Work out the finished part from the listing and answer in its coordinate system (mm). Round coordinates to 2 decimals unless told otherwise and drop trailing zeros. Loops run counter-clockwise (first coordinate to the right, second up) from the corner with the lowest first, then second, coordinate; pieces in that order, holes last. Notation, with made-up numbers: (8, 45) - (20, 45) arc R15 cw to (20, 66) - close; hole circle Ø1 at (72.25, 87). An arc over 180 degrees is marked (long way). Return JSON: item names as keys, results as strings.
from build123d import *

# Parameters (mm, degrees)
SKETCH1_R           = 4.2
BOSS_EXTRUDE1_DEPTH = 6.35


with BuildPart() as part:
    # Sketch1 → Boss-Extrude1 (new body)
    with BuildSketch(Plane(origin=(71.29240007, 0, 0), x_dir=(0, 0, -1), z_dir=(1, 0, 0))):
        with BuildLine():
            Line((916.713582015, 360.677443288), (922.204212824, 345.758563031))
            Line((922.204212824, 345.758563031), (895.973808013, 345.904541612))
            Line((895.973808013, 345.904541612), (897.39332308, 358.356278755))
            ThreePointArc((897.39332308, 358.356278755), (906.13613116, 367.152203744), (916.713582015, 360.677443288))
        make_face()
        with Locations((907.328968128, 357.223601629)):
            Circle(SKETCH1_R, mode=Mode.SUBTRACT)
    extrude(amount=BOSS_EXTRUDE1_DEPTH)


solid = part.part
1) Determine the mould class of faces 1 (the cylindrical face through (74.42, 353.5, -909.27)), 2 (the flat face through (74.42, 353.32, -919.42)), 3 (the flat face through (71.292, 352, -906)) for opening direction Y: pulls with the +Y half, pulls with the -Y half, needs draft (parallel to the pull), parting line crosses it, or undercut.
Verdict:
{"face 1": "undercut", "face 2": "pulls with the +Y half", "face 3": "needs draft"}
2) Flat-ended cylindrical pins translate along their axes: pin 1 (1 mm diameter, centred on x = 76, z = -908.5, fed in from +Y); pin 2 (1 mm diameter, centred on x = 72.5, y = 351, fed in from -Z); pin 3 (1 mm diameter, centred on x = 74, y = 355.5, fed in from +Z). Find the tip coordinate at first contact, or state that the pin passes through.
Verdict:
{"pin 1": "stops at y = 367.2", "pin 2": "stops at z = -920.46", "pin 3": "stops at z = -897.01"}
3) Section B-B (z = -906) is taken. Give the vertices of the cut face in (x, y).
Verdict:
{"outline": "(71.29, 345.85) - (77.64, 345.85) - (77.64, 353.24) - (71.29, 353.24) - close; (71.29, 361.21) - (77.64, 361.21) - (77.64, 367.13) - (71.29, 367.13) - close"}
4) Section C-C (x = 77.25) is taken. Give the vertices of the cut face in (y, z), and give its area (3 significant figures).
Verdict:
{"outline": "(345.76, -922.2) - (360.68, -916.71) arc R10 ccw to (358.36, -897.39) - (345.9, -895.97) - close; hole circle Ø8.4 at (357.22, -907.33)", "area": "370 mm2"}
5) Section D-D (y = 349.5) is taken. Give the vertices of the cut face in (x, z).
Verdict:
{"outline": "(71.29, -920.83) - (77.64, -920.83) - (77.64, -896.38) - (71.29, -896.38) - close"}
6) Find the intervals of material crossed by L1, parallel to Z at x = 75.5, y = 356.75; L2, parallel to Y at x = 73.25, z = -909; L3, parallel to Z at x = 76, y = 360.75, in increasing order.
Verdict:
{"L1": "z = -918.16 to -911.5, -903.16 to -897.21", "L2": "y = 345.83 to 353.37, 361.08 to 367.08", "L3": "z = -916.69 to -909.61, -905.05 to -897.97"}
7) Section A-A (y = 355.75) is taken. Give the vertices of the cut face in (x, z).
Verdict:
{"outline": "(71.29, -918.53) - (77.64, -918.53) - (77.64, -911.26) - (71.29, -911.26) - close; (71.29, -903.4) - (77.64, -903.4) - (77.64, -897.1) - (71.29, -897.1) - close"}
